```python
from build123d import *

# Parameters (mm, degrees)
EXTRUDE_2_DEPTH          = 20
SKETCH_3_R               = 1.65
CUT_EXTRUDE_1_DEPTH      = 126
CUT_EXTRUDE_1_DEPTH_BACK = 6
EXTRUDE_3_DEPTH          = 3
MIRROR_2_COPY_1_DEPTH    = 3
SKETCH_7_W               = 24
SKETCH_7_H               = 12
CUT_EXTRUDE_2_DEPTH      = 5
SKETCH_10_R              = 1
CUT_EXTRUDE_3_DEPTH      = 5


with BuildPart() as part:
    # 草图1 → 凸台-拉伸2 (new body)
    with BuildSketch(Plane.XY):
        Polygon((-65, 0), (65, 0), (65, -12), (60, -12), (60, -5), (-60, -5), (-60, -12), (-65, -12), align=None)
    extrude(amount=EXTRUDE_2_DEPTH)

    # 草图3 → 切除-拉伸1 (cut, two sides)
    with BuildSketch(Plane(origin=(-60, 0, 0), x_dir=(0, 0, -1), z_dir=(1, 0, 0))) as cut_extrude_1_sk:
        with Locations((-10, -9)):
            Circle(SKETCH_3_R)
    extrude(amount=CUT_EXTRUDE_1_DEPTH, mode=Mode.SUBTRACT)
    extrude(cut_extrude_1_sk.sketch, amount=-CUT_EXTRUDE_1_DEPTH_BACK, mode=Mode.SUBTRACT)

    # 草图4 → 凸台-拉伸3 (add)
    with BuildSketch(Plane(origin=(0, 0, 0), x_dir=(-1, 0, 0), z_dir=(0, 0, -1))):
        Polygon((54, -5), (60, -12), (60, -5), align=None)
    extrude_3 = extrude(amount=-EXTRUDE_3_DEPTH)

    # 镜向1: 凸台-拉伸3 across plane
    add(extrude_3.mirror(Plane.XY.offset(10)))

    # 镜向2: 凸台-拉伸3 across plane
    add(extrude_3.mirror(Plane(origin=(0, 0, 0), x_dir=(0, 0, 1), z_dir=(1, 0, 0))))

    # 镜向2 copy 1 sketch → 镜向2 copy 1 (add)
    with BuildSketch(Plane.XY.offset(20)):
        Polygon((54, -5), (60, -12), (60, -5), align=None)
    extrude(amount=-MIRROR_2_COPY_1_DEPTH)

    # 草图7 → 切除-拉伸2 (cut)
    with BuildSketch(Plane.XZ.offset(5)):
        with Locations((40, 10)):
            Rectangle(SKETCH_7_W, SKETCH_7_H)
    extrude(amount=-CUT_EXTRUDE_2_DEPTH, mode=Mode.SUBTRACT)

    # 草图10 → 切除-拉伸3 (cut)
    with BuildSketch(Plane.XZ.offset(5)):
        with Locations((53.835, 10)):
            Circle(SKETCH_10_R)
        with Locations((26.165, 10)):
            Circle(SKETCH_10_R)
    extrude(amount=-CUT_EXTRUDE_3_DEPTH, mode=Mode.SUBTRACT)


solid = part.part
```
Can you work these out from the model? Positions are in its coordinate system, mm. A direction names the side the tool comes from. Coordinates: 2 decimals unless noted, no trailing zeros. Loops run counter-clockwise (first coordinate to the right, second up) from the corner with the lowest first, then second, coordinate; pieces in that order, holes last. Notation, with made-up numbers: (-26.75, -4) - (-11.75, -4) arc R8 cw to (-11.75, 11) - close; hole circle Ø10 at (-12.5, -8.75). An arc over 180 degrees is marked (long way). Answer as CSV lines item,"result". Start each with the question number.
1) Which directions (+Z, -Z, +X, -X, +Y, -Y) give clear straight access to the entire face, cutting with the end or side of a thin tool? Please do faces 4 (the flat face through (58, -7, 3)), 5 (the flat face through (40, -3, 4)), 6 (the cylindrical face through (-62.465, -9.632, 8.476)), 7 (the flat face through (-57, -8.5, 1.5)).
2) Suppose I cut it at B-B (y = -9). Please give me the cut outline in (x, z), plus the area to 3 significant figures.
3) I need wall thicknesses on line 1 (X direction, y = -11.25, z = 5); line 2 (Y direction, x = -62.6, z = 10); line 3 (X direction, y = -4.75, z = 6.25). Which ranges of each line are inside material? Lowest first, please. Write a range as from..to.
4) For pin 1 (3 mm diameter, centred on y = -9, z = 10, fed in from -X); pin 2 (4 mm diameter, centred on x = -47, z = 12, fed in from -Y), each with a flat end and sliding along its axis, tell me the tip position at first contact or that it passes through.
5) Suppose I cut it at A-A (y = -1.25). Please give me the cut outline in (x, z) (3 decimals).
6) Suppose I cut it at C-C (x = -18). Please give me the cut outline in (y, z), plus the area to 3 significant figures.
7) Thinking about a two-plate mould opening in X: for faces 1 (the cylindrical face through (62.465, -9.632, 8.476)), 2 (the flat face through (65, -6, 10)), 3 (the flat face through (58, -7, 17)), which applies, pulls with the +X half, pulls with the -X half, needs draft (parallel to the pull), parting line crosses it, or undercut?
Check result:
1,face 4,"-Y"
1,face 5,"+Y, -Y"
1,face 6,"+X, -X"
1,face 7,"+Z, -Z, -Y"
2,outline,"(-65, 0) - (-57.43, 0) - (-57.43, 3) - (-60, 3) - (-60, 8.35) - (-65, 8.35) - close; (-65, 11.65) - (-60, 11.65) - (-60, 17) - (-57.43, 17) - (-57.43, 20) - (-65, 20) - close; (57.43, 0) - (65, 0) - (65, 8.35) - (60, 8.35) - (60, 3) - (57.43, 3) - close; (57.43, 17) - (60, 17) - (60, 11.65) - (65, 11.65) - (65, 20) - (57.43, 20) - close"
2,area,"198 mm²"
3,line 1,"x = -65..-60, 60..65"
3,line 2,"y = -12..-10.65, -7.35..0"
3,line 3,"x = -65..28, 52..65"
4,pin 1,"passes through"
4,pin 2,"stops at y = -5"
5,outline,"(-65, 0) - (65, 0) - (65, 20) - (-65, 20) - close; hole circle Ø2 at (26.165, 10); hole (28, 4) - (52, 4) - (52, 16) - (28, 16) - close; hole circle Ø2 at (53.835, 10)"
6,outline,"(-5, 0) - (0, 0) - (0, 20) - (-5, 20) - close"
6,area,"100 mm²"
7,face 1,"needs draft"
7,face 2,"pulls with the +X half"
7,face 3,"undercut"
